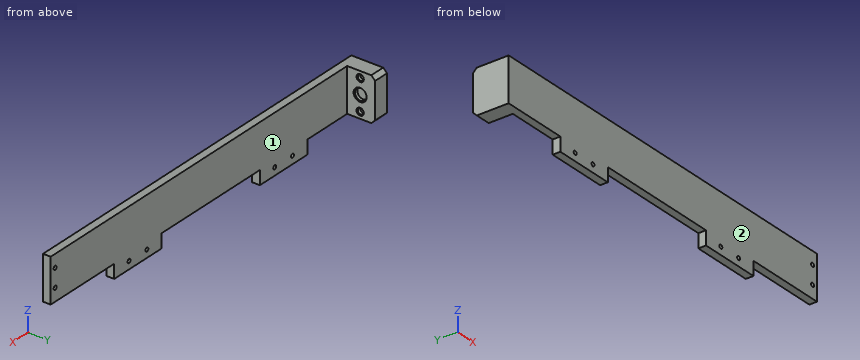
from build123d import *

# Parameters (mm, degrees)
SKETCH_1_W               = 211.216150174
SKETCH_1_H               = 56.943071366
EXTRUDE_1_DEPTH          = 20
SKETCH_2_W               = 1000
SKETCH_2_H               = 113.81790299
EXTRUDE_2_DEPTH          = 20
SKETCH_3_W               = 160
SKETCH_3_H               = 36.18209701
EXTRUDE_3_DEPTH          = 20
SKETCH_4_W               = 160
SKETCH_4_H               = 36.18209701
EXTRUDE_4_DEPTH          = 20
SKETCH_5_W               = 40
SKETCH_5_H               = 72.930561876
EXTRUDE_5_DEPTH          = 113.817902989
CUT_EXTRUDE_1_DEPTH      = 969.969572609
CUT_EXTRUDE_1_DEPTH_BACK = 10
SKETCH_6_R               = 15
SKETCH_6_R_2             = 7.5
SKETCH_7_W               = 113.81790299
SKETCH_7_H               = 20
EXTRUDE_6_DEPTH          = 40
CUT_EXTRUDE_2_DEPTH      = 553.797259551
CUT_EXTRUDE_2_DEPTH_BACK = 553.797259551
SKETCH_8_R               = 5
CHAMFER_1_SIZE           = 10
CHAMFER_2_SIZE           = 2
SKETCH_9_R               = 5
CUT_EXTRUDE_3_DEPTH      = 300


with BuildPart() as part:
    # 草图1 → 凸台-拉伸1 (new body)
    with BuildSketch(Plane(origin=(0, 0, 0), x_dir=(1, 0, 0), z_dir=(0, 1, 0))):
        Rectangle(SKETCH_1_W, SKETCH_1_H)
    extrude(amount=EXTRUDE_1_DEPTH)

    # 草图2 → 凸台-拉伸2 (add)
    with BuildSketch(Plane(origin=(0, 20, 0), x_dir=(1, 0, 0), z_dir=(0, 1, 0))):
        Rectangle(SKETCH_2_W, SKETCH_2_H)
    extrude(amount=-EXTRUDE_2_DEPTH)

    # 草图3 → 凸台-拉伸3 (add)
    with BuildSketch(Plane(origin=(0, 20, 0), x_dir=(1, 0, 0), z_dir=(0, 1, 0))):
        with Locations((-245.625, 75)):
            Rectangle(SKETCH_3_W, SKETCH_3_H)
    extrude(amount=-EXTRUDE_3_DEPTH)

    # 草图4 → 凸台-拉伸4 (add)
    with BuildSketch(Plane(origin=(0, 20, 0), x_dir=(1, 0, 0), z_dir=(0, 1, 0))):
        with Locations((245.625, 75)):
            Rectangle(SKETCH_4_W, SKETCH_4_H)
    extrude(amount=-EXTRUDE_4_DEPTH)

    # 草图5 → 凸台-拉伸5 (add)
    with BuildSketch(Plane.XY.offset(56.908951495)):
        with Locations((-480, 56.465280938)):
            Rectangle(SKETCH_5_W, SKETCH_5_H)
    extrude(amount=-EXTRUDE_5_DEPTH)

    # 草图6 → 切除-拉伸1 (cut, two sides: drawn at the far end of the back side and taken through both)
    with BuildSketch(Plane(origin=(-460, 0, 0), x_dir=(0, 0, -1), z_dir=(1, 0, 0)).offset(-CUT_EXTRUDE_1_DEPTH_BACK)):
        with Locations((0, 53.825309314)):
            Circle(SKETCH_6_R)
        with Locations((40, 53.825309314)):
            Circle(SKETCH_6_R_2)
        with Locations((-40, 53.825309314)):
            Circle(SKETCH_6_R_2)
    extrude(amount=CUT_EXTRUDE_1_DEPTH + CUT_EXTRUDE_1_DEPTH_BACK, mode=Mode.SUBTRACT)

    # 草图7 → 凸台-拉伸6 (add)
    with BuildSketch(Plane(origin=(500, 0, 0), x_dir=(0, 0, -1), z_dir=(1, 0, 0))):
        with Locations((0, 10)):
            Rectangle(SKETCH_7_W, SKETCH_7_H)
    extrude(amount=EXTRUDE_6_DEPTH)

    # 草图8 → 切除-拉伸2 (cut, two sides: drawn at the far end of the back side and taken through both)
    with BuildSketch(Plane(origin=(0, 20, 0), x_dir=(1, 0, 0), z_dir=(0, 1, 0)).offset(-CUT_EXTRUDE_2_DEPTH_BACK)):
        with Locations(Location((525, 23.75, 0), (0, 0, 270))):
            Circle(SKETCH_8_R)
        with Locations(Location((525, -23.75, 0), (0, 0, 270))):
            Circle(SKETCH_8_R)
    extrude(amount=CUT_EXTRUDE_2_DEPTH + CUT_EXTRUDE_2_DEPTH_BACK, mode=Mode.SUBTRACT)

    # 倒角1
    chamfer_1_edges = [part.edges().sort_by_distance(p)[0] for p in [
        (-480, 92.930561876, 56.908951495),
        (-480, 92.930561876, -56.908951494),
    ]]
    chamfer(chamfer_1_edges, length=CHAMFER_1_SIZE)

    # 倒角2
    chamfer_2_edges = [part.edges().sort_by_distance(p)[0] for p in [
        (-460, 53.825309314, 47.5),
        (-460, 53.825309314, -32.5),
        (-460, 53.825309314, 15),
    ]]
    chamfer(chamfer_2_edges, length=CHAMFER_2_SIZE)

    # 草图9 → 切除-拉伸3 (cut)
    with BuildSketch(Plane(origin=(0, 20, 0), x_dir=(1, 0, 0), z_dir=(0, 1, 0))):
        with Locations(Location((-275.625, 73.091048505, 0), (0, 0, 270))):
            Circle(SKETCH_9_R)
        with Locations(Location((-215.625, 73.091048505, 0), (0, 0, 270))):
            Circle(SKETCH_9_R)
        with Locations(Location((215.625, 73.091048505, 0), (0, 0, 270))):
            Circle(SKETCH_9_R)
        with Locations(Location((275.625, 73.091048505, 0), (0, 0, 270))):
            Circle(SKETCH_9_R)
    extrude(amount=-CUT_EXTRUDE_3_DEPTH, mode=Mode.SUBTRACT)


solid = part.part
Part model, mm, in its own coordinate system. Face numbers are marked on the shaded views. A direction names the side the tool comes from. Coordinates: 2 decimals unless noted, no trailing zeros. Loops run counter-clockwise (first coordinate to the right, second up) from the corner with the lowest first, then second, coordinate; pieces in that order, holes last. Notation, with made-up numbers: (-23.5, 5.5) - (-16.5, 5.5) arc R37 cw to (-16.5, 43.5) - close; hole circle Ø8 at (56.25, 63). An arc over 180 degrees is marked (long way). Write each question's results on one line, items separated by ' | '. Start each with the question number.
Q1. Probe line 1 along Z through (x, y) = (525, 15); line 2 along Y through (x, z) = (-466.5, 0); line 3 along X through (y, z) = (6, 23.75). List the from-to ranges inside material, lowest first.
Q2. Slice it at A-A on z = 0. Give the cut face in (x, y), and give its area (3 significant figures).
Q3. Slice it at B-B on x = 365. Give the cut face in (y, z), and give its area (3 significant figures).
Q4. Which spindle directions (+Z, -Z, +X, -X, +Y, -Y) get a long thin tool onto all of the face, cutting with end or side? Do the marked faces 1 and 2. Say none if no direction does.
Q5. Drop flat-ended pins along their axis: pin 1 Ø5 at (y, z) = (83.5, -11.5) entering from +X; pin 2 Ø6 at (y, z) = (14.5, -67.5) entering from +X (3 decimals); pin 3 Ø13 at (x, z) = (-215.62, -73.09) entering from +Y. Give the stop position or say it passes through.
Answer:
1) line 1: z = -56.91 to -28.75, -18.75 to 18.75, 28.75 to 56.91 | line 2: y = 0 to 38.83, 68.83 to 92.93 | line 3: x = -500 to 520, 530 to 540
2) outline: (-500, 0) - (540, 0) - (540, 20) - (-460, 20) - (-460, 36.83) - (-462, 38.83) - (-470, 38.83) - (-470, 68.83) - (-462, 68.83) - (-460, 70.83) - (-460, 92.93) - (-500, 92.93) - close | area: 23,400 mm2
3) outline: (0, -56.91) - (20, -56.91) - (20, 56.91) - (0, 56.91) - close | area: 2,280 mm2
4) face 1: +Z, -Z, +X, +Y | face 2: +Z, -Z, +X, -X, -Y
5) pin 1: stops at x = -460 | pin 2: stops at x = 325.625 | pin 3: stops at y = 20
